Here's how the part is built. I have some questions about the finished solid (model axes, mm). Give positions to 0.01 mm unless a question says otherwise; leave off trailing zeros. Write each loop counter-clockwise with the first axis right and the second up, starting at its lowest first coordinate (ties: lowest second). Pieces come first, ordered by that corner, then holes. Notation, with made-up numbers: (18.25, -17) -> (22.25, -17) arc R15 ccw to (22.25, -5) -> close; hole circle Ø5 at (-7.75, -36.5). An arc over 180 degrees is marked (long way). Use CSV: the item, a comma, the result in double quotes. Start each with the question number.
(1) Suppose I cut it at C-C on x = -1. List the corners of the cut face in (y, z) for me, plus the area to 3 significant figures.
(2) For pin 1 Ø12 at (y, z) = (15, 3.5) entering from -X; pin 2 Ø1 at (x, y) = (1.5, 21) entering from -Z; pin 3 Ø4 at (y, z) = (9.5, 6.5) entering from -X, each with a flat end and sliding along its axis, tell me the tip position at first contact or that it passes through.
(3) I need wall thicknesses on L1, parallel to X at y = 19.5, z = 8.25; L2, parallel to Z at x = 0.5, y = 22.25; L3, parallel to X at y = 11.5, z = 2. Which ranges of each line are inside material? Lowest first, please. Write a range as [from, to].
(4) Suppose I cut it at A-A on y = 22.5. List the corners of the cut face in (x, z) for me, plus the area to 3 significant figures.
(5) Suppose I cut it at B-B on z = 15.75. List the corners of the cut face in (x, y) for me, plus the area to 3 significant figures.
Autodesk Inventor part; units mm, degrees
ref_plane "YZ Plane" through (0, 0, 0) normal (1, 0, 0) x (0, 1, 0)
ref_plane "XZ Plane" through (0, 0, 0) normal (0, 1, 0) x (-1, 0, 0)
ref_plane "XY Plane" through (0, 0, 0) normal (0, 0, 1) x (1, 0, 0)
sketch "Sketch1" plane through (0, 0, 0) normal (0, 1, 0) x (-1, 0, 0)
  line L0 (7.2314, 12.2227) -> (8.6145, -3.2023)
  arc A0 (8.6145, -3.2023) -> (7.6223, -3.6232) centre (8.7714, -4.952) ccw
  line L1 (7.6223, -3.6232) -> (-3.1421, -6.1489)
  arc A1 (-8.374, -4.4651) -> (-3.1421, -6.1489) centre (-4.3594, -0.9611) ccw
  line L2 (-8.374, -4.4651) -> (-8.374, 9.8774)
  arc A2 (-7.4419, 14.0569) -> (-8.374, 9.8774) centre (1.4622, 9.8774) ccw
  line L3 (-7.4419, 14.0569) -> (-4.2604, 17.8775)
  arc A3 (-4.2604, 17.8775) -> (-2.3303, 17.8775) centre (-3.2954, 19.0365) ccw
  line L4 (-2.3303, 17.8775) -> (7.2314, 12.2227)
  point P0 (0, 0)
extrude "Extrusion1" add sketch "Sketch1" along normal blind 25.4
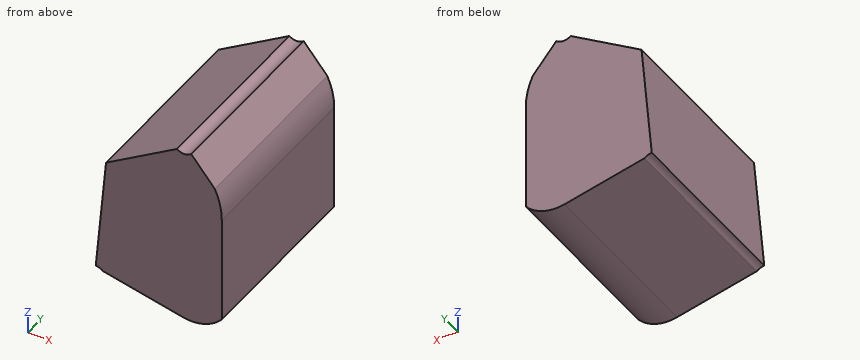
Geometry says:
1,outline,"(0, -5.18) -> (25.4, -5.18) -> (25.4, 15.91) -> (0, 15.91) -> close"
1,area,"536 mm²"
2,pin 1,"x = -8.55"
2,pin 2,"z = -5.88"
2,pin 3,"x = -7.92"
3,L1,"[-7.59, 8.37]"
3,L2,"[-5.53, 16.8]"
3,L3,"[-8.15, 8.37]"
4,outline,"(-8.61, -3.2) arc R1.76 cw to (-7.62, -3.62) -> (3.14, -6.15) arc R5.33 ccw to (8.37, -4.47) -> (8.37, 9.88) arc R9.84 ccw to (7.44, 14.06) -> (4.26, 17.88) arc R1.51 cw to (2.33, 17.88) -> (-7.23, 12.22) -> close"
4,area,"333 mm²"
5,outline,"(-1.27, 0) -> (6.03, 0) -> (6.03, 25.4) -> (-1.27, 25.4) -> close"
5,area,"185 mm²"
